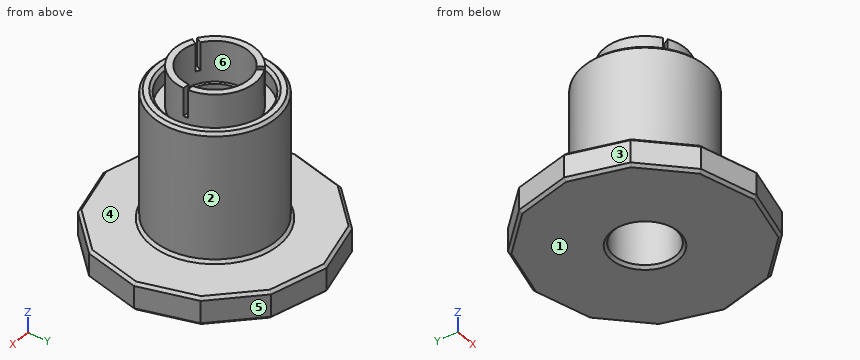
```python
from build123d import *

# Parameters (mm, degrees)
SKETCH_R             = 14.5
SKETCH_R_2           = 12.1
PAD_DEPTH            = 14.6
SKETCH001_W          = 30.380329
SKETCH001_H          = 1.5
POCKET_DEPTH         = 97.067871
POLARPATTERN_COUNT   = 3
SKETCH003_R          = 22
PAD001_DEPTH         = 40
SKETCH004_R          = 22
SKETCH004_R_2        = 18.1
PAD002_DEPTH         = 6
PAD003_DEPTH         = 10
SKETCH005_R          = 11
POCKET001_DEPTH      = 50.001
POCKET001_DEPTH_BACK = 14.601
CHAMFER_SIZE         = 1


with BuildPart() as part:
    # Sketch → Pad (new body)
    with BuildSketch(Plane.XY):
        Circle(SKETCH_R)
        Circle(SKETCH_R_2, mode=Mode.SUBTRACT)
    extrude(amount=PAD_DEPTH)

    # Sketch001 → Pocket (cut, through all)
    with BuildSketch(Plane.XY.offset(4.6)):
        with Locations((15.190164, 0)):
            Rectangle(SKETCH001_W, SKETCH001_H)
    pocket = extrude(amount=POCKET_DEPTH, mode=Mode.SUBTRACT)

    # PolarPattern: Pocket ×3 about axis
    polarpattern_axis = Axis((0, 0, 4.6), (0, 0, 1))
    for i in range(1, POLARPATTERN_COUNT):
        add(pocket.rotate(polarpattern_axis, i * 360 / POLARPATTERN_COUNT), mode=Mode.SUBTRACT)

    # Sketch003 → Pad001 (join)
    with BuildSketch(Plane.XY):
        Circle(SKETCH003_R)
    extrude(amount=-PAD001_DEPTH)

    # Sketch004 → Pad002 (join)
    with BuildSketch(Plane.XY):
        Circle(SKETCH004_R)
        Circle(SKETCH004_R_2, mode=Mode.SUBTRACT)
    extrude(amount=PAD002_DEPTH)

    # Sketch002 → Pad003 (join)
    with BuildSketch(Plane.XY.offset(-40)):
        Polygon((20, -34.641016), (34.641016, -20), (40, 0), (34.641016, 20), (20, 34.641016), (0, 40), (-20, 34.641016), (-34.641016, 20), (-40, 0), (-34.641016, -20), (-20, -34.641016), (0, -40), align=None)
    extrude(amount=-PAD003_DEPTH)

    # Sketch005 → Pocket001 (cut, two sides)
    with BuildSketch(Plane.XY) as pocket001_sk:
        Circle(SKETCH005_R)
    extrude(amount=-POCKET001_DEPTH, mode=Mode.SUBTRACT)
    extrude(pocket001_sk.sketch, amount=POCKET001_DEPTH_BACK, mode=Mode.SUBTRACT)

    # Chamfer
    chamfer_edges = [part.edges().sort_by_distance(p)[0] for p in [
        (27.320508, -27.320508, -50),
        (10, -37.320508, -50),
        (37.320508, -10, -50),
        (-10, -37.320508, -50),
        (37.320508, 10, -50),
        (-27.320508, -27.320508, -50),
        (27.320508, 27.320508, -50),
        (-37.320508, -10, -50),
        (10, 37.320508, -50),
        (-37.320508, 10, -50),
        (-10, 37.320508, -50),
        (-27.320508, 27.320508, -50),
        (-11, 0, -50),
        (27.320508, -27.320508, -40),
        (10, -37.320508, -40),
        (37.320508, -10, -40),
        (-10, -37.320508, -40),
        (37.320508, 10, -40),
        (-27.320508, -27.320508, -40),
        (27.320508, 27.320508, -40),
        (-37.320508, -10, -40),
        (10, 37.320508, -40),
        (-37.320508, 10, -40),
        (-10, 37.320508, -40),
        (-27.320508, 27.320508, -40),
        (-22, 0, -40),
        (-22, 0, 6),
        (-18.1, 0, 6),
    ]]
    chamfer(chamfer_edges, length=CHAMFER_SIZE)


solid = part.part
```
The model under review builds one solid part; all positions refer to its coordinate system, in mm. Face numbers are marked on the shaded views. A direction names the side the tool comes from. Round coordinates to 2 decimals unless told otherwise and drop trailing zeros. Loops run counter-clockwise (first coordinate to the right, second up) from the corner with the lowest first, then second, coordinate; pieces in that order, holes last. Notation, with made-up numbers: (71.5, 12) -> (82.5, 12) arc R30 ccw to (82.5, 47) -> close; hole circle Ø9 at (4.25, 15). An arc over 180 degrees is marked (long way). Answer as a JSON object with one key per item and string values. Group by question number.
1) For the marked faces 1 and 2, list the 3-axis set-ups (+Z, -Z, +X, -X, +Y, -Y) from which the entire face can be reached by the end or side of a thin tool; tool diameter is ignored.
2) We need section B-B on z = -43. Write out the cut boundary in (x, y).
3) For pin 1 Ø2.5 at (x, z) = (13, 12) entering from +Y; pin 2 Ø8 at (x, z) = (11, -43) entering from -Y; pin 3 Ø6 at (y, z) = (18.5, -39) entering from -X, all flat-tipped, find the tip position at first contact; note any pin that passes through.
4) We need section A-A on z = 11.5. Write out the cut boundary in (x, y), then the cut area to 3 significant figures.
5) For line 1 (Y direction, x = 0, z = 1); line 2 (Y direction, x = 0, z = 10.5); line 3 (Y direction, x = 0, z = -32.5), list the stretches that pass through material, from the lowest coordinate up. Write a range as [from, to].
6) Mouldability with a two-part tool opening along X and no side actions: class the marked faces 3, 4, 5 and 6 as released by +X, released by -X, zero draft, split by the parting line, or undercut.
7) We need section D-D on z = -32. Write out the cut boundary in (x, y).
8) We need section C-C on x = -26. Write out the cut boundary in (y, z).
Result set:
{
 "1": {"face 1": "-Z, +X, -X, +Y, -Y", "face 2": "+Z"},
 "2": {"outline": "(-40, 0) -> (-34.64, -20) -> (-20, -34.64) -> (0, -40) -> (20, -34.64) -> (34.64, -20) -> (40, 0) -> (34.64, 20) -> (20, 34.64) -> (0, 40) -> (-20, 34.64) -> (-34.64, 20) -> close; hole circle Ø22 at (0, 0)"},
 "3": {"pin 1": "y = 8.5", "pin 2": "y = -38.12", "pin 3": "x = -35.64"},
 "4": {"outline": "(-7.89, -12.17) -> (-6.69, -10.08) arc R12.1 cw to (-6.69, 10.08) -> (-7.89, 12.17) arc R14.5 ccw to start; (-6.59, -12.92) arc R14.5 ccw to (14.48, -0.75) -> (12.08, -0.75) arc R12.1 cw to (-5.39, -10.83) -> close; (-6.59, 12.92) -> (-5.39, 10.83) arc R12.1 cw to (12.08, 0.75) -> (14.48, 0.75) arc R14.5 ccw to start", "area": "190 mm²"},
 "5": {"line 1": "[-22, -18.1], [-14.5, -12.1], [12.1, 14.5], [18.1, 22]", "line 2": "[-14.5, -12.1], [12.1, 14.5]", "line 3": "[-22, -11], [11, 22]"},
 "6": {"face 3": "released by -X", "face 4": "zero draft", "face 5": "released by +X", "face 6": "undercut"},
 "7": {"outline": "circle Ø44 at (0, 0); hole circle Ø22 at (0, 0)"},
 "8": {"outline": "(-28.64, -49) -> (-27.23, -50) -> (27.23, -50) -> (28.64, -49) -> (28.64, -41) -> (27.23, -40) -> (-27.23, -40) -> (-28.64, -41) -> close"}
}
